Geometry: final body of the model. Coordinates: model frame, mm. Face numbers are marked on the shaded views. Give positions to 0.01 mm unless a question says otherwise; leave off trailing zeros. Order: outer loops, then holes, each group sorted by start corner. A loop starts at its lowest first (then second) coordinate and runs counter-clockwise, first axis right, second up. Notation, with made-up numbers: (71, -4) -> (101, -4) arc R22 ccw to (101, 23) -> close; hole circle Ø11 at (7.25, -19.5). An arc over 180 degrees is marked (long way). Answer in a Markdown table with one row per item. Add a question column.
Q1. Cut plane A-A on x = 0. Return the cut outline in (y, z), and give its area (3 significant figures).
Q2. Line query: line 1 along Y through (x, z) = (0, 3.6); line 2 along Y through (x, z) = (30, 4.25). Output: solid intervals per line, ascending. Write a range as from..to.
Q3. Contact query for flat-ended pins moving along their axis: P1, Ø2, axis at x = 2.5, z = 3, coming from the -Y side; P2, Ø1.5, axis at y = 30.5, z = 0.5, coming from the +X side. Output: stop coordinate, or through.
Q4. Pull-direction query (Y, two-part tool) for the marked faces 1 and 2; classes: +Y half, -Y half, draft (parallel to the pull), parting line (faces both ways), or undercut.
Autodesk Inventor part; units mm, degrees
ref_plane "YZ Plane" through (0, 0, 0) normal (1, 0, 0) x (0, 1, 0)
ref_plane "XZ Plane" through (0, 0, 0) normal (0, 1, 0) x (-1, 0, 0)
ref_plane "XY Plane" through (0, 0, 0) normal (0, 0, 1) x (1, 0, 0)
sketch "Эскиз1" plane through (0, 0, 0) normal (0, 0, 1) x (1, 0, 0)
  circle A0 centre (0, 0) radius 30
  circle A1 centre (0, 0) radius 45
  dimension "d0" = 60
  dimension "d1" = 90
extrude "Выдавливание1" add sketch "Эскиз1" along normal blind 5
sketch "Эскиз2" plane through (0, 0, 0) normal (1, 0, 0) x (0, 1, 0)
  line L0 (-45, 0) -> (-45, 5)
  line L1 (0, -0.8) -> (0, 4.8)
  line L2 (-45, 0) -> (-45, 5)
  line L3 (-45, 2.5) -> (-44, 2.5)
  circle A0 centre (-44, 2.5) radius 1
  line L4 (-44, 3.5) -> (-45, 3.5)
  line L5 (-44, 1.5) -> (-45, 1.5)
  line L6 (-45, 0) -> (-45, 5)
  point P0 (0, 0)
  dimension "d6" = 1
  dimension "d7" = 2
revolve "Вращение1" cut sketch "Эскиз2" angle 360 about axis through (0, 0, -10) along (0, 0, 1)
sketch "Эскиз3" plane through (0, 0, 0) normal (1, 0, 0) x (0, 1, 0)
  line L0 (45, 0) -> (-45, 0)
  line L1 (0, -4) -> (0, 6.5)
  line L2 (33.2404, 3.2596) -> (36.5, 0)
  line L3 (45, 5) -> (-45, 5)
  line L4 (33.2404, 3.2596) -> (33.2404, 5)
  line L5 (30, 5) -> (30, 0)
  point P0 (0, 0)
  dimension "d13" = 45
revolve "Вращение2" cut sketch "Эскиз3" angle 360 about axis through (0, 0, -10) along (0, 0, 1) contours L0 L5 L3 L4 L2
properties part number "Кольцо сальника 2" material "Сталь, легированная"
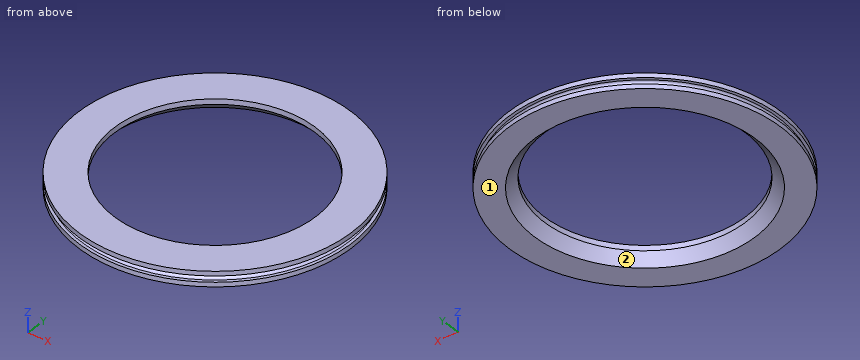
Completed:
| question | item | result |
|---|---|---|
| 1 | outline | (-45, 0) -> (-36.5, 0) -> (-33.24, 3.26) -> (-33.24, 5) -> (-45, 5) -> (-45, 3.5) -> (-44, 3.5) arc R1 cw to (-44, 1.5) -> (-45, 1.5) -> close; (33.24, 3.26) -> (36.5, 0) -> (45, 0) -> (45, 1.5) -> (44, 1.5) arc R1 cw to (44, 3.5) -> (45, 3.5) -> (45, 5) -> (33.24, 5) -> close |
| 1 | area | 99.8 mm² |
| 2 | line 1 | y = -45..-33.24, 33.24..45 |
| 2 | line 2 | y = -33.54..-14.32, 14.32..33.54 |
| 3 | P1 | stops at y = -44.97 |
| 3 | P2 | stops at x = 33.76 |
| 4 | face 1 | draft |
| 4 | face 2 | undercut |
